The listing builds one solid part. Answer for the finished solid, in the listing's coordinates (mm). Face numbers are marked on the shaded views. A direction names the side the tool comes from. Give positions to 0.01 mm unless a question says otherwise; leave off trailing zeros. Loops run counter-clockwise (first coordinate to the right, second up) from the corner with the lowest first, then second, coordinate; pieces in that order, holes last. Notation, with made-up numbers: (40.5, 81) - (53.5, 81) arc R10 cw to (53.5, 85) - close; hole circle Ø6 at (50, 85). An arc over 180 degrees is marked (long way). Write each question's results on one line, items separated by ' | '.
from build123d import *

# Parameters (mm, degrees)
SKETCH1_W           = 55.61
SKETCH1_H           = 8
SKETCH1_R           = 2.75
BOSS_EXTRUDE1_DEPTH = 22
SKETCH2_W           = 5
SKETCH2_H           = 5
BOSS_EXTRUDE2_DEPTH = 30
BOSS_EXTRUDE3_DEPTH = 5
FILLET1_R           = 3


with BuildPart() as part:
    # Sketch1 → Boss-Extrude1 (new body)
    with BuildSketch(Plane(origin=(0, 0, 0), x_dir=(1, 0, 0), z_dir=(0, 1, 0))):
        with Locations((27.805, 4)):
            Rectangle(SKETCH1_W, SKETCH1_H)
        with Locations(Location((27.805, 4, 0), (0, 0, 270))):
            Circle(SKETCH1_R, mode=Mode.SUBTRACT)
        with Locations(Location((10.575, 4, 0), (0, 0, 270))):
            Circle(SKETCH1_R, mode=Mode.SUBTRACT)
        with Locations(Location((45.035, 4, 0), (0, 0, 270))):
            Circle(SKETCH1_R, mode=Mode.SUBTRACT)
    extrude(amount=BOSS_EXTRUDE1_DEPTH)

    # Sketch2 → Boss-Extrude2 (add)
    with BuildSketch(Plane.XY):
        with Locations((25.305, 19.5)):
            Rectangle(SKETCH2_W, SKETCH2_H)
        with Locations((30.305, 19.5)):
            Rectangle(SKETCH2_W, SKETCH2_H)
    extrude(amount=BOSS_EXTRUDE2_DEPTH)

    # Sketch3 → Boss-Extrude3 (add)
    with BuildSketch(Plane(origin=(0, 22, 0), x_dir=(1, 0, 0), z_dir=(0, 1, 0))):
        with BuildLine():
            Line((22.805, -30), (32.805, -30))
            ThreePointArc((32.805, -30), (27.805, -35), (22.805, -30))
        make_face()
    extrude(amount=-BOSS_EXTRUDE3_DEPTH)

    # Fillet1
    fillet1_edges = [part.edges().sort_by_distance(p)[0] for p in [
        (55.61, 22, -4),
        (22.805, 19.5, 0),
        (32.805, 19.5, 0),
        (0, 22, -4),
    ]]
    fillet(fillet1_edges, radius=FILLET1_R)


solid = part.part
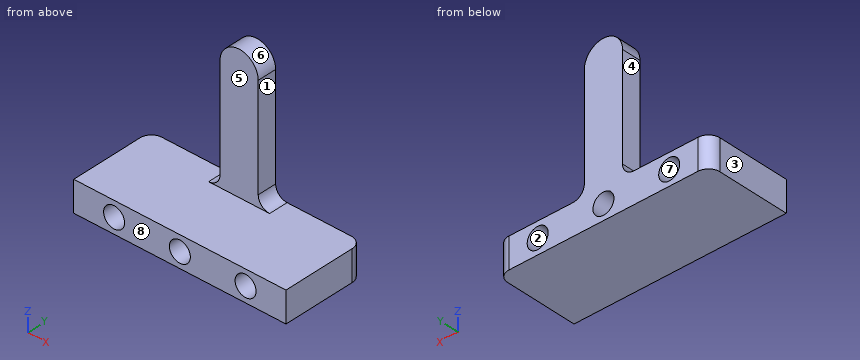
Item 1: A cutting plane is placed at D-D, the plane z = 8. Determine the outline of the cut face in (x, y) (3 decimals).
Values found:
outline: (22.805, 17) - (32.805, 17) - (32.805, 22) - (22.805, 22) - close
Item 2: Find the intervals of material crossed by line 1 along X through (y, z) = (5.25, -4) (3 decimals); line 2 along X through (y, z) = (18, -2.5); line 3 along Z through (x, y) = (3.5, 15), in increasing order. Write a range as [from, to].
Values found:
line 1: x = [0, 7.825], [13.325, 25.055], [30.555, 42.285], [47.785, 55.61] | line 2: x = [0, 8.27], [12.88, 25.5], [30.11, 42.73], [47.34, 55.61] | line 3: z = [-8, 0]
Item 3: A cutting plane is placed at C-C, the plane x = 6.5. Determine the outline of the cut face in (y, z).
Values found:
outline: (0, -8) - (22, -8) - (22, 0) - (0, 0) - close
Item 4: A cutting plane is placed at B-B, the plane y = 3.75. Determine the outline of the cut face in (x, z) (3 decimals), plus the area to 3 significant figures.
Values found:
outline: (0, -8) - (55.61, -8) - (55.61, 0) - (0, 0) - close; hole circle Ø5.5 at (10.575, -4); hole circle Ø5.5 at (27.805, -4); hole circle Ø5.5 at (45.035, -4) | area: 374 mm²
Item 5: Flat-ended cylindrical pins translate along their axes: P1, Ø4, axis at y = 18.5, z = 23, coming from the -X side (3 decimals); P2, Ø8, axis at x = 16, z = 16, coming from the -Y side; P3, Ø4, axis at y = 20, z = 15, coming from the +X side (3 decimals); P4, Ø1, axis at x = 11.5, y = 13.5, coming from the +Z side. Find the tip coordinate at first contact, or state that the pin passes through.
Values found:
P1: stops at x = 22.805 | P2: passes through | P3: stops at x = 32.805 | P4: stops at z = 0
Item 6: For the marked faces 1, 2, 3, 4 and 5, determine the directions among +Z, -Z, +X, -X, +Y, -Y from which every point of the face is accessible in a straight line to the end or side of a thin tool.
Values found:
face 1: +Z, +X, +Y, -Y | face 2: +Y, -Y | face 3: +Z, -Z, -X, +Y, -Y | face 4: +Z, -X, +Y, -Y | face 5: +Z, +X, -X, -Y
Item 7: A cutting plane is placed at A-A, the plane z = -4. Determine the outline of the cut face in (x, y) (3 decimals).
Values found:
outline: (0, 0) - (7.825, 0) - (7.825, 22) - (3, 22) arc R3 ccw to (0, 19) - close; (13.325, 0) - (25.055, 0) - (25.055, 22) - (13.325, 22) - close; (30.555, 0) - (42.285, 0) - (42.285, 22) - (30.555, 22) - close; (47.785, 0) - (55.61, 0) - (55.61, 19) arc R3 ccw to (52.61, 22) - (47.785, 22) - close
Item 8: For a pull along X with two mould halves and no side action, classify the marked faces 6, 7 and 8 as released by +X, released by -X, zero draft, split by the parting line, or undercut.
Values found:
face 6: split by the parting line | face 7: undercut | face 8: zero draft
